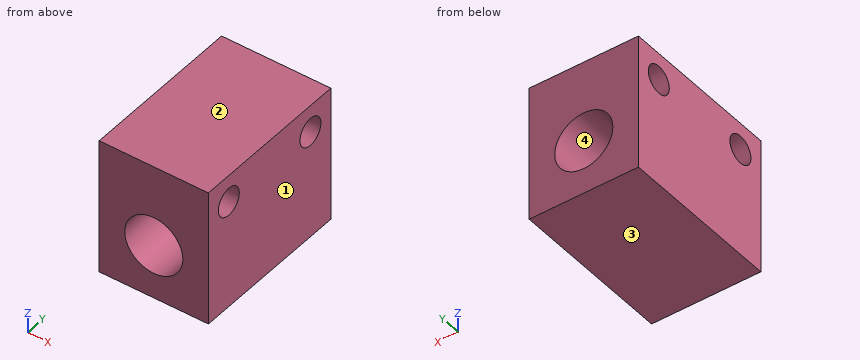
from build123d import *

# Parameters (mm, degrees)
SKETCH1_W               = 12.7
SKETCH1_H               = 19.05
BOSS_EXTRUDE1_DEPTH     = 15.875
F_1_4_CLEARANCE_HOLE1_D = 6.7564
F_4_CLEARANCE_HOLE1_D   = 3.2639


with BuildPart() as part:
    # Sketch1 → Boss-Extrude1 (new body)
    with BuildSketch(Plane.XY):
        Rectangle(SKETCH1_W, SKETCH1_H)
    extrude(amount=BOSS_EXTRUDE1_DEPTH)

    # 1/4 Clearance Hole1 (through all)
    with Locations(Plane(origin=(0, 9.525, 0), x_dir=(1, 0, 0), z_dir=(0, 1, 0))):
        with Locations((0, -6.35)):
            Hole(F_1_4_CLEARANCE_HOLE1_D / 2)

    # #4 Clearance Hole1 (through all)
    with Locations(Plane(origin=(6.35, 0, 0), x_dir=(0, 0, -1), z_dir=(1, 0, 0))):
        with Locations((-12.7, 6.35), (-12.7, -6.35)):
            Hole(F_4_CLEARANCE_HOLE1_D / 2)


solid = part.part
CAD build for the part. Positions are in the model's coordinates, mm. Face numbers are marked on the shaded views. Round coordinates to 2 decimals unless told otherwise and drop trailing zeros. Loops run counter-clockwise (first coordinate to the right, second up) from the corner with the lowest first, then second, coordinate; pieces in that order, holes last. Notation, with made-up numbers: (23, 37.5) - (65, 37.5) arc R19 cw to (65, 70.5) - close; hole circle Ø1 at (61.5, -14.5). An arc over 180 degrees is marked (long way). Put each result on its own line as item: value.
1. Two-plate mould, pull along Z, no slides. Class the marked faces 1, 2, 3 and 4: released by +Z, released by -Z, zero draft, split by the parting line, or undercut.
Geometry check:
face 1: zero draft
face 2: released by +Z
face 3: released by -Z
face 4: undercut
2. Slice it at A-A on x = 0. List the corners of the cut face in (y, z) (3 decimals), and give its area (3 significant figures).
Geometry check:
outline: (-9.525, 0) - (9.525, 0) - (9.525, 2.972) - (-9.525, 2.972) - close; (-9.525, 9.728) - (9.525, 9.728) - (9.525, 15.875) - (-9.525, 15.875) - close; hole circle Ø3.264 at (-6.35, 12.7); hole circle Ø3.264 at (6.35, 12.7)
area: 157 mm²
3. Slice it at C-C on z = 6.35. List the corners of the cut face in (x, y) (3 decimals).
Geometry check:
outline: (-6.35, -9.525) - (-3.378, -9.525) - (-3.378, 9.525) - (-6.35, 9.525) - close; (3.378, -9.525) - (6.35, -9.525) - (6.35, 9.525) - (3.378, 9.525) - close
4. Slice it at B-B on y = 6.35. List the corners of the cut face in (x, z) (3 decimals).
Geometry check:
outline: (-6.35, 0) - (6.35, 0) - (6.35, 11.068) - (-6.35, 11.068) - close; (-6.35, 14.332) - (6.35, 14.332) - (6.35, 15.875) - (-6.35, 15.875) - close; hole circle Ø6.756 at (0, 6.35)
5. Pin check, flat tip, straight feed: P1, Ø2, axis at y = -6.35, z = 12.7, coming from the -X side. Stop position of the tip, or through.
Geometry check:
P1: through
6. Wall check: line 1 (Y direction, x = 0.25, z = 12.7) (3 decimals); line 2 (Z direction, x = 0, y = -2.75) (3 decimals); line 3 (Z direction, x = -0.5, y = 6.75) (3 decimals). Give the ranges that are in metal, low to high.
Geometry check:
line 1: -9.525 to -7.982, -4.718 to 4.718, 7.982 to 9.525
line 2: 0 to 2.972, 9.728 to 15.875
line 3: 0 to 3.009, 9.691 to 11.118, 14.282 to 15.875
7. Slice it at D-D on z = 13.5. List the corners of the cut face in (x, y) (3 decimals).
Geometry check:
outline: (-6.35, -9.525) - (6.35, -9.525) - (6.35, -7.772) - (-6.35, -7.772) - close; (-6.35, -4.928) - (6.35, -4.928) - (6.35, 4.928) - (-6.35, 4.928) - close; (-6.35, 7.772) - (6.35, 7.772) - (6.35, 9.525) - (-6.35, 9.525) - close
